```python
from build123d import *

# Parameters (mm, degrees)
SKETCH1_W           = 50
SKETCH1_H           = 30
SKETCH1_R           = 2
SKETCH1_R_2         = 2.5
BOSS_EXTRUDE1_DEPTH = 2
SKETCH2_R           = 5
SKETCH2_R_2         = 2.5
BOSS_EXTRUDE2_DEPTH = 14.75
SKETCH3_R           = 3.5
SKETCH3_R_2         = 2.5
BOSS_EXTRUDE3_DEPTH = 0.5
SKETCH4_R           = 3.5
SKETCH4_R_2         = 2.5
BOSS_EXTRUDE4_DEPTH = 0.5
BOSS_EXTRUDE5_DEPTH = 14.75


with BuildPart() as part:
    # Sketch1 → Boss-Extrude1 (new body)
    with BuildSketch(Plane(origin=(0, 0, 0), x_dir=(1, 0, 0), z_dir=(0, 1, 0))):
        with Locations((25, 15)):
            Rectangle(SKETCH1_W, SKETCH1_H)
        with Locations(Location((5, 15, 0), (0, 0, 270))):
            Circle(SKETCH1_R, mode=Mode.SUBTRACT)
        with Locations(Location((45, 15, 0), (0, 0, 270))):
            Circle(SKETCH1_R, mode=Mode.SUBTRACT)
        with Locations(Location((17.5, 15, 0), (0, 0, 270))):
            Circle(SKETCH1_R_2, mode=Mode.SUBTRACT)
        with Locations(Location((32.5, 15, 0), (0, 0, 270))):
            Circle(SKETCH1_R_2, mode=Mode.SUBTRACT)
    extrude(amount=BOSS_EXTRUDE1_DEPTH)

    # Sketch2 → Boss-Extrude2 (add)
    with BuildSketch(Plane(origin=(0, 2, 0), x_dir=(1, 0, 0), z_dir=(0, 1, 0))):
        with Locations(Location((32.5, 15, 0), (0, 0, 90))):
            Circle(SKETCH2_R)
        with Locations(Location((32.5, 15, 0), (0, 0, 270))):
            Circle(SKETCH2_R_2, mode=Mode.SUBTRACT)
    extrude(amount=BOSS_EXTRUDE2_DEPTH)

    # Sketch3 → Boss-Extrude3 (add)
    with BuildSketch(Plane(origin=(0, 2, 0), x_dir=(1, 0, 0), z_dir=(0, 1, 0))):
        with Locations(Location((17.5, 15, 0), (0, 0, 90))):
            Circle(SKETCH3_R)
        with Locations(Location((17.5, 15, 0), (0, 0, 270))):
            Circle(SKETCH3_R_2, mode=Mode.SUBTRACT)
    extrude(amount=BOSS_EXTRUDE3_DEPTH)

    # Sketch4 → Boss-Extrude4 (add)
    with BuildSketch(Plane(origin=(0, 16.75, 0), x_dir=(1, 0, 0), z_dir=(0, 1, 0))):
        with Locations(Location((32.5, 15, 0), (0, 0, 270))):
            Circle(SKETCH4_R)
        with Locations(Location((32.5, 15, 0), (0, 0, 270))):
            Circle(SKETCH4_R_2, mode=Mode.SUBTRACT)
    extrude(amount=BOSS_EXTRUDE4_DEPTH)

    # Sketch5 → Boss-Extrude5 (add)
    with BuildSketch(Plane(origin=(0, 2, 0), x_dir=(1, 0, 0), z_dir=(0, 1, 0))):
        with BuildLine():
            Line((50, 30), (28.200775839, 30))
            Line((28.200775839, 30), (28.200775839, 17.552777235))
            ThreePointArc((28.200775839, 17.552777235), (33.823608551, 19.821624249), (37.5, 15))
            ThreePointArc((37.5, 15), (33.823608551, 10.178375751), (28.200775839, 12.447222765))
            Line((28.200775839, 12.447222765), (28.200775839, 0))
            Line((28.200775839, 0), (50, 0))
            Line((50, 0), (39.100387919, 15))
            Line((39.100387919, 15), (50, 30))
        make_face()
    extrude(amount=BOSS_EXTRUDE5_DEPTH)


solid = part.part
```
Verification items for the finished model (mm, model axes). A direction names the side the tool comes from. Give positions to 0.01 mm unless a question says otherwise; leave off trailing zeros. Loops run counter-clockwise (first coordinate to the right, second up) from the corner with the lowest first, then second, coordinate; pieces in that order, holes last. Notation, with made-up numbers: M 79.5,81.5 L 83.5,81.5 A18 ccw 83.5,103.5 Z; hole C 78.25,10.5 d8. An arc over 180 degrees is marked long. Return JSON: item names as keys, results as strings.
1) Tool access check on faces 1 (the flat face through (50, 1, -15)), 2 (the flat face through (44.474, 9.272, -22.395)), 3 (the cylindrical face through (36, 17, -15)), 4 (the flat face through (15, 2.5, -14)), 5 (the cylindrical face through (34, 9, -17)). Record the directions out of +Z, -Z, +X, -X, +Y, -Y that give a thin tool (end or side, any length) a straight path to the whole face; none if there is none.
Findings:
{"face 1": "+Z, -Z, +X, +Y, -Y", "face 2": "+X, +Y", "face 3": "+Y", "face 4": "+Z, -Z, -X, +Y", "face 5": "+Y, -Y"}
2) Section check B-B, the plane z = -16.25. Count the separate pieces of the cut face and the enclosed holes in it, and give its area (3 significant figures).
Findings:
{"separate pieces": "5", "enclosed holes": "0", "area": "191 mm2"}
3) Section check A-A, the plane x = 32.5. Enter the section's corners in (y, z).
Findings:
{"outline": "M 0,-30 L 16.75,-30 L 16.75,-18.5 L 17.25,-18.5 L 17.25,-17.5 L 0,-17.5 Z; M 0,-12.5 L 17.25,-12.5 L 17.25,-11.5 L 16.75,-11.5 L 16.75,0 L 0,0 Z"}
4) Material ranges on L1, parallel to X at y = 1.35, z = -15; L2, parallel to Y at x = 44, z = -6.75; L3, parallel to Y at x = 12.5, z = -22, recorded low to high. Write a range as [from, to].
Findings:
{"L1": "x = [0, 3], [7, 15], [20, 30], [35, 43], [47, 50]", "L2": "y = [0, 16.75]", "L3": "y = [0, 2]"}
5) Section check C-C, the plane y = 14.25. Enter the section's corners in (x, z).
Findings:
{"outline": "M 28.2,-30 L 50,-30 L 39.1,-15 L 50,0 L 28.2,0 L 28.2,-12.45 A5 ccw 28.2,-17.55 Z; hole C 32.5,-15 d5"}
6) Section check D-D, the plane x = 17.5. Enter the section's corners in (y, z).
Findings:
{"outline": "M 0,-30 L 2,-30 L 2,-18.5 L 2.5,-18.5 L 2.5,-17.5 L 0,-17.5 Z; M 0,-12.5 L 2.5,-12.5 L 2.5,-11.5 L 2,-11.5 L 2,0 L 0,0 Z"}
7) Mould release check, pull along X, two halves, no side actions. Record for faces 6 (the flat face through (0, 1, -15)), 7 (the cylindrical face through (43, 1, -15)), 8 (the flat face through (36, 8, -30)), 9 (the cylindrical face through (19, 1, -17)): released by +X, released by -X, zero draft, split by the parting line, or undercut.
Findings:
{"face 6": "released by -X", "face 7": "undercut", "face 8": "zero draft", "face 9": "undercut"}
8) Gauge pin test, flat ends, axial feed: P1, Ø1.5, axis at y = 14.5, z = -8.5, coming from the -X side; P2, Ø6.5, axis at x = 45, z = -15, coming from the +Y side; P3, Ø14, axis at x = 14.5, z = -15, coming from the +Y side. Record the tip position at first contact, or that the pin passes through.
Findings:
{"P1": "stops at x = 28.2", "P2": "stops at y = 2", "P3": "stops at y = 2.5"}
